The listing builds one solid part. Answer for the finished solid, in the listing's coordinates (mm). A direction names the side the tool comes from. Give positions to 0.01 mm unless a question says otherwise; leave off trailing zeros. Order: outer loops, then holes, each group sorted by start corner. A loop starts at its lowest first (then second) coordinate and runs counter-clockwise, first axis right, second up. Notation, with made-up numbers: (6, 55.25) - (46, 55.25) arc R28 cw to (46, 93.25) - close; hole circle Ø10 at (12.25, 47). An arc over 180 degrees is marked (long way). Write each question's results on one line, items separated by ' | '. Start each with the question number.
1. Section C-C (y = 10.5) is taken. Give the vertices of the cut face in (x, z).
2. Section B-B (z = 0) is taken. Give the vertices of the cut face in (x, y), and give its area (3 significant figures).
3. Determine the mould class of faces 3 (the face through (5, 0, 17)), 4 (the face through (16.453, 5.916, 5.181)), 5 (the face through (-20, -12, 0)), 6 (the face through (0, 0, -22)) for opening direction Z: released by +Z, released by -Z, zero draft, split by the parting line, or undercut.
4. Find the intervals of material crossed by L1, parallel to Z at x = 0, y = -8.25; L2, parallel to Z at x = 0, y = 7.5; L3, parallel to X at y = 11, z = -12.5, in increasing order.
5. Which of the six approach directions +Z, -Z, +X, -X, +Y, -Y give full straight-line access (tool end or side, diameter ignored) to faces 1 (the face through (-4.01, -5.92, -18.06)), 2 (the face through (-22, 0, 0))?
6. Section D-D (y = -4.5) is taken. Give the vertices of the cut face in (x, z), and give its area (3 significant figures).
7. Section A-A (x = 0) is taken. Give the vertices of the cut face in (y, z).
from build123d import *

# Parameters (mm, degrees)
F0_W     = 44
F0_H     = 44
F0_R     = 18.5
F1_DEPTH = 12
F2_W     = 44
F2_H     = 44
F2_R     = 17.25
F3_DEPTH = 12


# Not quite as in the source:
# - a feature names something its author has since deleted; it is built from what else it names


with BuildPart() as f1:
    # F0 (on Front) → F1 (new body)
    with BuildSketch(Plane.XZ):
        Rectangle(F0_W, F0_H)
        Circle(F0_R, mode=Mode.SUBTRACT)
    extrude(amount=F1_DEPTH)

    # F2 (on Front) → F3 (join)
    with BuildSketch(Plane.XZ):
        Rectangle(F2_W, F2_H)
        Circle(F2_R, mode=Mode.SUBTRACT)
    extrude(amount=-F3_DEPTH)


solid = f1.part
Reported:
1) outline: (-22, -22) - (22, -22) - (22, 22) - (-22, 22) - close; hole circle Ø34.5 at (0, 0)
2) outline: (-22, -12) - (-18.5, -12) - (-18.5, 0) - (-17.25, 0) - (-17.25, 12) - (-22, 12) - close; (17.25, 0) - (18.5, 0) - (18.5, -12) - (22, -12) - (22, 12) - (17.25, 12) - close | area: 198 mm²
3) face 3: undercut | face 4: undercut | face 5: zero draft | face 6: released by -Z
4) L1: -22 to -18.5, 18.5 to 22 | L2: -22 to -17.25, 17.25 to 22 | L3: -22 to -11.89, 11.89 to 22
5) face 1: -Y | face 2: +Z, -Z, -X, +Y, -Y
6) outline: (-22, -22) - (22, -22) - (22, 22) - (-22, 22) - close; hole circle Ø37 at (0, 0) | area: 861 mm²
7) outline: (-12, -22) - (12, -22) - (12, -17.25) - (0, -17.25) - (0, -18.5) - (-12, -18.5) - close; (-12, 18.5) - (0, 18.5) - (0, 17.25) - (12, 17.25) - (12, 22) - (-12, 22) - close
